Input: part model. Units: mm. Frame: model coordinates. A direction names the side the tool comes from. Give positions to 0.01 mm unless a question says otherwise; leave off trailing zeros. Write each loop counter-clockwise with the first axis right and the second up, starting at its lowest first coordinate (ties: lowest second). Pieces come first, ordered by that corner, then holes. Notation, with made-up numbers: (-28.5, -28) -> (-12.5, -28) arc R32 cw to (-12.5, 1) -> close; hole circle Ø2 at (65, -18.75). An arc over 180 degrees is marked (long way). Return JSON: item names as keys, results as strings. Group by question number.
Item 1: Set-up query: faces 5 (the face through (0, 6, 17.8)), 6 (the face through (-3.75, 1, 15)), 7 (the face through (0, 0, 15)). Return all of +Z, -Z, +X, -X, +Y, -Y with unobstructed straight access to the full face (end or side cutting, diameter ignored); none if empty.
Item 2: Section C-C, the plane x = 0. Return loops of the section in (y, z), then the cut area to 3 significant figures.
Item 3: Section A-A, the plane z = 8. Return loops of the section in (x, y).
Item 4: Line query: line 1 (Z direction, x = 0, y = 1.4); line 2 (Z direction, x = 0.75, y = 4.5); line 3 (X direction, y = 3.75, z = 5.5). Output: solid intervals per line, ascending. Write a range as [from, to].
Item 5: Section B-B, the plane y = 7.5. Return loops of the section in (x, z).
Item 6: Mould query, pull axis X, two halves, no side actions, for faces 1 (the face through (6, 2.2, 15)), 2 (the face through (0, 6, 26.2)), 3 (the face through (-7.9, 3, 15)), 4 (the face through (3.75, 1, 15)). Classes: released by +X, released by -X, zero draft, split by the parting line, or undercut.
Item 7: Section D-D, the plane z = 17.5. Return loops of the section in (x, y).
Item 8: Pin query (flat end, axial travel): P1, Ø1.3, axis at y = 5, z = 6.5, coming from the +X side; P2, Ø6.5, axis at x = 0, z = 22, coming from the +Y side; P3, Ø1.1, axis at y = 1, z = 12.5, coming from the +X side. Return the tip coordinate at first contact, or that it passes through.
from build123d import *

# Parameters (mm, degrees)
PAD003_DEPTH           = 30
SKETCH005_W            = 8.4
SKETCH005_H            = 8.4
POCKET001_DEPTH        = 4.5
LINEARPATTERN002_COUNT = 2
LINEARPATTERN002_PITCH = 14
SKETCH004_R            = 2.75
HOLE001_DEPTH          = 25
LINEARPATTERN003_COUNT = 2
LINEARPATTERN003_PITCH = 14


with BuildPart() as part:
    # Sketch006 → Pad003 (new body)
    with BuildSketch(Plane.XY):
        Polygon((0, 0), (0, 8), (-4, 8), (-7.9, 4.1), (-7.9, 2.2), (-3.75, 2.2), (-3.75, 0), align=None)
    pad003 = extrude(amount=PAD003_DEPTH)

    # Mirrored001: Pad003 across Sketch006 V_Axis
    add(pad003.mirror(Plane(origin=(0, 0, 0), x_dir=(0, 0, 1), z_dir=(1, 0, 0))))

    # Sketch005 (on DatumPlane) → Pocket001 (cut)
    with BuildSketch(Plane(origin=(0, 8, 0), x_dir=(-1, 0, 0), z_dir=(0, 1, 0))):
        with Locations((0, 8)):
            Rectangle(SKETCH005_W, SKETCH005_H)
    pocket001 = extrude(amount=-POCKET001_DEPTH, mode=Mode.SUBTRACT)

    # LinearPattern002: Pocket001 ×2
    with Locations(*[(0, 0, i * LINEARPATTERN002_PITCH) for i in range(1, LINEARPATTERN002_COUNT)]):
        add(pocket001, mode=Mode.SUBTRACT)

    # Sketch004 (on DatumPlane) → Hole001 (cut)
    with BuildSketch(Plane(origin=(0, 8, 0), x_dir=(-1, 0, 0), z_dir=(0, 1, 0))):
        with Locations((0, 8)):
            Circle(SKETCH004_R)
    hole001 = extrude(amount=-HOLE001_DEPTH, mode=Mode.SUBTRACT)

    # LinearPattern003: Hole001 ×2
    with Locations(*[(0, 0, i * LINEARPATTERN003_PITCH) for i in range(1, LINEARPATTERN003_COUNT)]):
        add(hole001, mode=Mode.SUBTRACT)


solid = part.part
Answer below:
{
 "1": {"face 5": "+Y", "face 6": "+Z, -Z, -X, -Y", "face 7": "+Z, -Z, +X, -X, -Y"},
 "2": {"outline": "(0, 0) -> (8, 0) -> (8, 3.8) -> (3.5, 3.8) -> (3.5, 5.25) -> (0, 5.25) -> close; (0, 10.75) -> (3.5, 10.75) -> (3.5, 12.2) -> (8, 12.2) -> (8, 17.8) -> (3.5, 17.8) -> (3.5, 19.25) -> (0, 19.25) -> close; (0, 24.75) -> (3.5, 24.75) -> (3.5, 26.2) -> (8, 26.2) -> (8, 30) -> (0, 30) -> close", "area": "126 mm2"},
 "3": {"outline": "(-7.9, 2.2) -> (-3.75, 2.2) -> (-3.75, 0) -> (-2.75, 0) -> (-2.75, 3.5) -> (-4.2, 3.5) -> (-4.2, 7.8) -> (-7.9, 4.1) -> close; (2.75, 0) -> (3.75, 0) -> (3.75, 2.2) -> (7.9, 2.2) -> (7.9, 4.1) -> (4.2, 7.8) -> (4.2, 3.5) -> (2.75, 3.5) -> close"},
 "4": {"line 1": "z = [0, 5.25], [10.75, 19.25], [24.75, 30]", "line 2": "z = [0, 3.8], [12.2, 17.8], [26.2, 30]", "line 3": "x = [-7.9, -4.2], [4.2, 7.9]"},
 "5": {"outline": "(-4.5, 0) -> (4.5, 0) -> (4.5, 30) -> (-4.5, 30) -> close; hole (-4.2, 3.8) -> (4.2, 3.8) -> (4.2, 12.2) -> (-4.2, 12.2) -> close; hole (-4.2, 17.8) -> (4.2, 17.8) -> (4.2, 26.2) -> (-4.2, 26.2) -> close"},
 "6": {"face 1": "zero draft", "face 2": "undercut", "face 3": "released by -X", "face 4": "released by +X"},
 "7": {"outline": "(-7.9, 2.2) -> (-3.75, 2.2) -> (-3.75, 0) -> (3.75, 0) -> (3.75, 2.2) -> (7.9, 2.2) -> (7.9, 4.1) -> (4, 8) -> (-4, 8) -> (-7.9, 4.1) -> close"},
 "8": {"P1": "stops at x = 7.65", "P2": "stops at y = 3.5", "P3": "stops at x = 3.75"}
}
